Geometry: final body of the model. Coordinates: model frame, mm. A direction names the side the tool comes from. Give positions to 0.01 mm unless a question says otherwise; leave off trailing zeros. Write each loop counter-clockwise with the first axis right and the second up, starting at its lowest first coordinate (ties: lowest second). Pieces come first, ordered by that corner, then holes. Notation, with made-up numbers: M 54,47.25 L 112,47.25 A10 ccw 112,63.25 Z; hole C 11,-32.75 d10. An arc over 180 degrees is marked long. Use a Markdown table: item, result. Add a question column.
1) Pin query (flat end, axial travel): pin 1 (3 mm diameter, centred on x = -19, y = 19, fed in from -Z); pin 2 (5 mm diameter, centred on x = 19, y = 19, fed in from +Z); pin 3 (6 mm diameter, centred on x = 19.5, y = 10, fed in from +Z). Return the tip coordinate at first contact, or that it passes through.
2) Set-up query: faces 1 (the flat face through (0, 14, 7)), 2 (the flat face through (-17, -21, 7)), 3 (the cylindrical face through (19, 21, 3)). Return all of +Z, -Z, +X, -X, +Y, -Y with unobstructed straight access to the full face (end or side cutting, diameter ignored); none if empty.
3) Line query: line 1 (Y direction, x = -19, z = 4); line 2 (Y direction, x = -19, z = 8.45); line 3 (X direction, y = -18, z = 1). Output: solid intervals per line, ascending.
4) Section C-C on x = -19. Return the cut outline in (y, z), then the cut area to 3 significant figures.
5) Section A-A on y = -19. Return the cut outline in (x, z), then the cut area to 3 significant figures.
6) Section B-B on z = 10.5. Return the cut outline in (x, y), then the cut area to 3 significant figures.
7) Draft query along Y for faces 4 (the flat face through (0, -25.6, 6)), 5 (the flat face through (0, 20, 12)), 6 (the cylindrical face through (-17.12, 21.95, 9.46)). Return one class per face: +Y half, -Y half, draft (parallel to the pull), parting line (faces both ways), or undercut.
8) Section D-D on x = 12. Return the cut outline in (y, z).
```python
from build123d import *

# Parameters (mm, degrees)
F0_W     = 51.2
F0_H     = 11.6
F0_R     = 2
F0_H_2   = 28
F1_DEPTH = 2
F2_W     = 51.2
F2_H     = 11.6
F2_R     = 2
F3_DEPTH = 5
F4_W     = 51.2
F4_H     = 11.6
F4_R     = 3.5
F5_DEPTH = 5


with BuildPart() as f1:
    # F0 (on Top) → F1 (new body)
    with BuildSketch(Plane.XY):
        with Locations((0, -19.8)):
            Rectangle(F0_W, F0_H)
        with Locations((-19, -19)):
            Circle(F0_R, mode=Mode.SUBTRACT)
        with Locations((19, -19)):
            Circle(F0_R, mode=Mode.SUBTRACT)
        Rectangle(F0_W, F0_H_2)
        with Locations((0, 19.8)):
            Rectangle(F0_W, F0_H)
        with Locations((-19, 19)):
            Circle(F0_R, mode=Mode.SUBTRACT)
        with Locations((19, 19)):
            Circle(F0_R, mode=Mode.SUBTRACT)
    extrude(amount=F1_DEPTH)

    # F2 (on face) → F3 (join)
    with BuildSketch(Plane.XY.offset(2)):
        with Locations((0, 19.8)):
            Rectangle(F2_W, F2_H)
        with Locations((-19, 19)):
            Circle(F2_R, mode=Mode.SUBTRACT)
        with Locations((19, 19)):
            Circle(F2_R, mode=Mode.SUBTRACT)
        with Locations((0, -19.8)):
            Rectangle(F2_W, F2_H)
        with Locations((-19, -19)):
            Circle(F2_R, mode=Mode.SUBTRACT)
        with Locations((19, -19)):
            Circle(F2_R, mode=Mode.SUBTRACT)
    extrude(amount=F3_DEPTH)

    # F4 (on face) → F5 (join)
    with BuildSketch(Plane.XY.offset(7)):
        with Locations((0, 19.8)):
            Rectangle(F4_W, F4_H)
        with Locations((-19, 19)):
            Circle(F4_R, mode=Mode.SUBTRACT)
        with Locations((19, 19)):
            Circle(F4_R, mode=Mode.SUBTRACT)
        with Locations((0, -19.8)):
            Rectangle(F4_W, F4_H)
        with Locations((-19, -19)):
            Circle(F4_R, mode=Mode.SUBTRACT)
        with Locations((19, -19)):
            Circle(F4_R, mode=Mode.SUBTRACT)
    extrude(amount=F5_DEPTH)


solid = f1.part
```
Found:
| question | item | result |
|---|---|---|
| 1 | pin 1 | through |
| 1 | pin 2 | z = 7 |
| 1 | pin 3 | z = 2 |
| 2 | face 1 | +Z, +X, -X |
| 2 | face 2 | +Z |
| 2 | face 3 | +Z, -Z |
| 3 | line 1 | -25.6 to -21, -17 to -14, 14 to 17, 21 to 25.6 |
| 3 | line 2 | -25.6 to -22.5, -15.5 to -14, 14 to 15.5, 22.5 to 25.6 |
| 3 | line 3 | -25.6 to -20.73, -17.27 to 17.27, 20.73 to 25.6 |
| 4 | outline | M -25.6,0 L -21,0 L -21,7 L -22.5,7 L -22.5,12 L -25.6,12 Z; M -17,0 L 17,0 L 17,7 L 15.5,7 L 15.5,12 L 14,12 L 14,2 L -14,2 L -14,12 L -15.5,12 L -15.5,7 L -17,7 Z; M 21,0 L 25.6,0 L 25.6,12 L 22.5,12 L 22.5,7 L 21,7 Z |
| 4 | area | 208 mm² |
| 5 | outline | M -25.6,0 L -21,0 L -21,7 L -22.5,7 L -22.5,12 L -25.6,12 Z; M -17,0 L 17,0 L 17,7 L 15.5,7 L 15.5,12 L -15.5,12 L -15.5,7 L -17,7 Z; M 21,0 L 25.6,0 L 25.6,12 L 22.5,12 L 22.5,7 L 21,7 Z |
| 5 | area | 488 mm² |
| 6 | outline | M -25.6,-25.6 L 25.6,-25.6 L 25.6,-14 L -25.6,-14 Z; M -25.6,14 L 25.6,14 L 25.6,25.6 L -25.6,25.6 Z; hole C -19,-19 d7; hole C -19,19 d7; hole C 19,-19 d7; hole C 19,19 d7 |
| 6 | area | 1,030 mm² |
| 7 | face 4 | -Y half |
| 7 | face 5 | draft |
| 7 | face 6 | undercut |
| 8 | outline | M -25.6,0 L 25.6,0 L 25.6,12 L 14,12 L 14,2 L -14,2 L -14,12 L -25.6,12 Z |
